Could you check a few things on this model? Use its own coordinates, in mm. A direction names the side the tool comes from. Round coordinates to 2 decimals unless told otherwise and drop trailing zeros. Order: outer loops, then holes, each group sorted by start corner. A loop starts at its lowest first (then second) coordinate and runs counter-clockwise, first axis right, second up.
```python
from build123d import *

# Parameters (mm, degrees)
SKETCH028_W             = 27
SKETCH028_H             = 6.22
SKETCH028_R             = 1.75
PAD016_DEPTH            = 4.5
SKETCH029_W             = 4.1
SKETCH029_H             = 6.22
PAD017_DEPTH            = 8.4
SKETCH030_W             = 12.25
SKETCH030_H             = 6
PAD018_DEPTH            = 15
BODY004_PLACEMENT_ANGLE = 90


with BuildPart() as obj1:
    # Sketch028 → Pad016 (new body)
    with BuildSketch(Plane.XY):
        Rectangle(SKETCH028_W, SKETCH028_H)
        with Locations((10.75, 0)):
            Circle(SKETCH028_R, mode=Mode.SUBTRACT)
        with Locations((-10.75, 0)):
            Circle(SKETCH028_R, mode=Mode.SUBTRACT)
    extrude(amount=PAD016_DEPTH)

    # Sketch029 (on Face7 of Pad016) → Pad017 (join)
    with BuildSketch(Plane(origin=(0, 0, 0), x_dir=(1, 0, 0), z_dir=(0, 0, -1))):
        with Locations((-5, 0)):
            Rectangle(SKETCH029_W, SKETCH029_H)
        with Locations((5, 0)):
            Rectangle(SKETCH029_W, SKETCH029_H)
    extrude(amount=PAD017_DEPTH)

    # Sketch030 (on Face10 of Pad017) → Pad018 (join)
    with BuildSketch(Plane.XZ.offset(3.11)):
        with Locations((0, 5.85)):
            Rectangle(SKETCH030_W, SKETCH030_H)
    extrude(amount=PAD018_DEPTH)


with BuildPart() as obj1_1:
    # Body004 placement: moved
    add(obj1.part.moved(Location((-20, 23, -4.5))).rotate(Axis((-20, 23, -4.5), (0, 0, -1)), BODY004_PLACEMENT_ANGLE))


with BuildPart() as part_mirroring002:
    # Part__Mirroring002: instance of obj1
    add(obj1_1.part.mirror(Plane(origin=(0, 0, 0), x_dir=(1, 0, 0), z_dir=(0, 1, 0))))


solid = part_mirroring002.part
```
Q1. I need wall thicknesses on L1, parallel to X at y = -33.75, z = -3.6; L2, parallel to Y at x = -18, z = -9.25; L3, parallel to Z at x = -33.5, y = -24. Which ranges of each line are inside material? Lowest first, please.
Q2. For P1, Ø1.9, axis at x = -19.5, y = -28, coming from the +Z side; P2, Ø1.9, axis at x = -21, y = -13.5, coming from the -Z side; P3, Ø3, axis at x = -35.5, z = -4, coming from the +Y side; P4, Ø3.5, axis at y = -21, z = 3, coming from the +X side, each with a flat end and sliding along its axis, tell me the tip position at first contact or that it passes through.
Q3. Imagine slicing it at B-B, the plane x = -20. Please give me the cut outline in (y, z), then the cut area to 3 significant figures.
Q4. For faces 1 (the flat face through (-20, -30.05, -9)), 2 (the flat face through (-20, -14.2, -4.5)), 3 (the flat face through (-20, -25.95, -9)), 4 (the flat face through (-20, -23, 0)), 5 (the flat face through (-31, -29.125, 1)), which set-ups out of +Z, -Z, +X, -X, +Y, -Y let a thin tool reach every point of the face, with its end or its side?
Q5. Imagine slicing it at D-D, the plane z = -3. Please give me the cut outline in (x, y), then the cut area to 3 significant figures.
Q6. Imagine slicing it at C-C, the plane z = -6.25. Please give me the cut outline in (x, y).
Q7. Imagine slicing it at A-A, the plane y = -12.25. Please give me the cut outline in (x, z), then the cut area to 3 significant figures.
Filled in:
1. L1: x = -23.11 to -21.75, -18.25 to -16.89
1. L2: y = -30.05 to -25.95, -20.05 to -15.95
1. L3: z = -1.65 to 4.35
2. P1: stops at z = 0
2. P2: stops at z = -4.5
2. P3: passes through
2. P4: stops at x = -23.11
3. outline: (-36.5, -4.5) - (-35.5, -4.5) - (-35.5, 0) - (-36.5, 0) - close; (-32, -4.5) - (-30.05, -4.5) - (-30.05, -12.9) - (-25.95, -12.9) - (-25.95, -4.5) - (-20.05, -4.5) - (-20.05, -12.9) - (-15.95, -12.9) - (-15.95, -4.5) - (-14, -4.5) - (-14, 0) - (-32, 0) - close; (-10.5, -4.5) - (-9.5, -4.5) - (-9.5, 0) - (-10.5, 0) - close
3. area: 159 mm2
4. face 1: -Z, +X, -X, -Y
4. face 2: -Z, +X, -X, +Y
4. face 3: -Z, +X, -X
4. face 4: +Z, +X, +Y, -Y
4. face 5: +Z, -Z, -X, -Y
5. outline: (-23.11, -36.5) - (-16.89, -36.5) - (-16.89, -9.5) - (-23.11, -9.5) - close; hole circle Ø3.5 at (-20, -33.75); hole circle Ø3.5 at (-20, -12.25)
5. area: 149 mm2
6. outline: (-23.11, -30.05) - (-16.89, -30.05) - (-16.89, -25.95) - (-23.11, -25.95) - close; (-23.11, -20.05) - (-16.89, -20.05) - (-16.89, -15.95) - (-23.11, -15.95) - close
7. outline: (-23.11, -4.5) - (-21.75, -4.5) - (-21.75, 0) - (-23.11, 0) - close; (-18.25, -4.5) - (-16.89, -4.5) - (-16.89, 0) - (-18.25, 0) - close
7. area: 12.2 mm2
